Here's how the part is built. I have some questions about the finished solid (model axes, mm). Face numbers are marked on the shaded views. A direction names the side the tool comes from. Round coordinates to 2 decimals unless told otherwise and drop trailing zeros. Order: outer loops, then holes, each group sorted by start corner. A loop starts at its lowest first (then second) coordinate and runs counter-clockwise, first axis right, second up. Notation, with made-up numbers: (-30.5, 22.25) - (4.5, 22.25) arc R26 cw to (4.5, 52.25) - close; hole circle Ø10 at (-24, 38). An arc over 180 degrees is marked (long way). Answer as a JSON object with one key per item and string values.
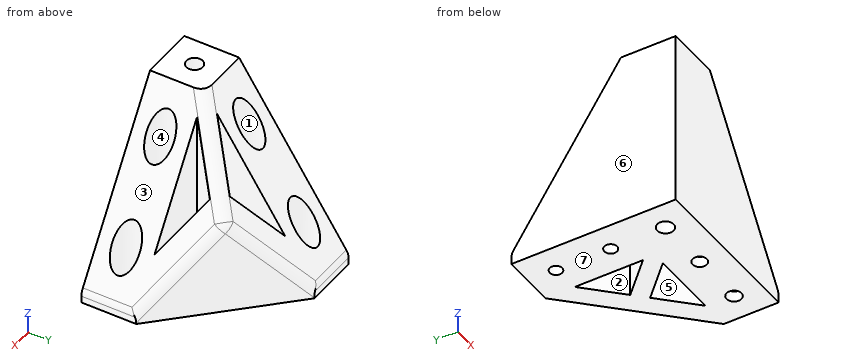
```python
from build123d import *

# Parameters (mm, degrees)
F1_DEPTH  = 65
F3_DEPTH  = 60.001
F5_DEPTH  = 60.001
F6_R      = 2.5
F6_R_2    = 2.6062767238
F6_R_3    = 2.7274571226
F6_R_4    = 2.3400008441
F6_R_5    = 2.2698965194
F7_DEPTH  = 65.001
F8_R      = 5
F9_DEPTH  = 61
F10_R     = 5
F11_R     = 3
F12_DEPTH = 65.001


with BuildPart() as f1:
    # F0 (on Top) → F1 (new body)
    with BuildSketch(Plane.XY):
        Polygon((0, 60), (0, 0), (60, 0), (60, 20), (20, 60), align=None)
        Polygon((49.3933982822, 20), (24.4768448174, 20), (36.9351215498, 32.4582767324), align=None, mode=Mode.SUBTRACT)
        Polygon((32.4582767324, 36.9351215498), (20, 24.4768448174), (20, 49.3933982822), align=None, mode=Mode.SUBTRACT)
    extrude(amount=F1_DEPTH)

    # F2 (on face) → F3 (cut, through all)
    with BuildSketch(Plane.XZ):
        Polygon((60, 65), (20, 65), (60, 4), align=None)
    extrude(amount=-F3_DEPTH, mode=Mode.SUBTRACT)

    # F4 (on face) → F5 (cut, through all)
    with BuildSketch(Plane(origin=(0, 0, 0), x_dir=(0, -1, 0), z_dir=(-1, 0, 0))):
        Polygon((-60, 65), (-60, 4), (-20, 65), align=None)
    extrude(amount=-F5_DEPTH, mode=Mode.SUBTRACT)

    # F6 (on face) → F7 (cut, through all)
    with BuildSketch(Plane(origin=(0, 0, 0), x_dir=(1, 0, 0), z_dir=(0, 0, -1))):
        with Locations((10, -10)):
            Circle(F6_R)
        with Locations((30, -10)):
            Circle(F6_R_2)
        with Locations((50, -10)):
            Circle(F6_R_3)
        with Locations((10, -30)):
            Circle(F6_R_4)
        with Locations((10, -50)):
            Circle(F6_R_5)
    extrude(amount=-F7_DEPTH, mode=Mode.SUBTRACT)

    # F8 (on face) → F9 (cut)
    with BuildSketch(Plane.XY.offset(65)):
        with Locations((30, 10)):
            Circle(F8_R)
        with Locations((50, 10)):
            Circle(F8_R)
        with Locations((10, 30)):
            Circle(F8_R)
        with Locations((10, 50)):
            Circle(F8_R)
    extrude(amount=-F9_DEPTH, mode=Mode.SUBTRACT)

    # F10
    f10_edges = [f1.edges().sort_by_distance(p)[0] for p in [
        (50, 30, 19.25),
        (30, 50, 19.25),
        (60, 10, 4),
        (10, 60, 4),
        (30, 30, 49.75),
    ]]
    fillet(f10_edges, radius=F10_R)

    # F11 (on face) → F12 (cut, through all)
    with BuildSketch(Plane(origin=(0, 0, 0), x_dir=(1, 0, 0), z_dir=(0, 0, -1))):
        with Locations((10, -10)):
            Circle(F11_R)
    extrude(amount=-F12_DEPTH, mode=Mode.SUBTRACT)


solid = f1.part
```
1. If I drill on L1, parallel to X at y = 10, z = 1.05; L2, parallel to Y at x = 10, z = 1.4; L3, parallel to Y at x = 10, z = 20.75, over which ranges is the centre line in solid material (lowest first)? Write a range as [from, to].
Responses:
{"L1": "[0, 7], [13, 27.39], [32.61, 47.27], [52.73, 60]", "L2": "[0, 7], [13, 27.66], [32.34, 47.73], [52.27, 60]", "L3": "[0, 7], [13, 25], [35, 45]"}
2. Imagine slicing it at B-B (x = 10). List the corners of the cut face in (y, z) for me (3 decimals), plus the area to 3 significant figures.
Responses:
{"outline": "(0, 0) - (7, 0) - (7, 65) - (0, 65) - close; (13, 0) - (27.66, 0) - (27.66, 4) - (25, 4) - (25, 57.375) - (20, 65) - (13, 65) - close; (32.34, 0) - (47.73, 0) - (47.73, 4) - (45, 4) - (45, 26.875) - (35, 42.125) - (35, 4) - (32.34, 4) - close; (52.27, 0) - (60, 0) - (60, 2.507) arc R5 ccw to (59.181, 5.249) - (55, 11.625) - (55, 4) - (52.27, 4) - close", "area": "1,640 mm2"}
3. Thinking about a two-plate mould opening in X: for the marked faces 4, 5, 6 and 7, which applies, pulls with the +X half, pulls with the -X half, needs draft (parallel to the pull), parting line crosses it, or undercut?
Responses:
{"face 4": "undercut", "face 5": "undercut", "face 6": "pulls with the -X half", "face 7": "needs draft"}
4. Imagine slicing it at A-A (y = 9). List the corners of the cut face in (x, z) for me.
Responses:
{"outline": "(0, 0) - (7.17, 0) - (7.17, 65) - (0, 65) - close; (12.83, 0) - (27.59, 0) - (27.59, 4) - (25.1, 4) - (25.1, 57.22) - (20, 65) - (12.83, 65) - close; (32.41, 0) - (47.46, 0) - (47.46, 4) - (45.1, 4) - (45.1, 26.72) - (34.9, 42.28) - (34.9, 4) - (32.41, 4) - close; (52.54, 0) - (60, 0) - (60, 2.51) arc R5 ccw to (59.18, 5.25) - (54.9, 11.78) - (54.9, 4) - (52.54, 4) - close"}
5. Imagine slicing it at C-C (z = 24). Give the number of separate pieces and of enclosed holes in the cut face, plus the area to 3 significant figures.
Responses:
{"separate pieces": "1", "enclosed holes": "3", "area": "1,590 mm2"}
6. For P1, Ø16, axis at x = 30, y = 10, coming from the +Z side; P2, Ø5, axis at y = 15.5, z = 45, coming from the +X side; P3, Ø11, axis at x = 11, y = 50.5, coming from the +Z side (3 decimals); P4, Ø5, axis at x = 12.5, y = 25, coming from the -Z side, each with a flat end and sliding along its axis, tell me the tip position at first contact or that it passes through.
Responses:
{"P1": "z = 61.95", "P2": "x = 34.75", "P3": "z = 26.875", "P4": "z = 0"}
7. For the marked faces 1, 2 and 3, which set-ups out of +Z, -Z, +X, -X, +Y, -Y let a thin tool reach every point of the face, with its end or its side?
Responses:
{"face 1": "+Z", "face 2": "+Z, -Z", "face 3": "+Z, +X, +Y, -Y"}
